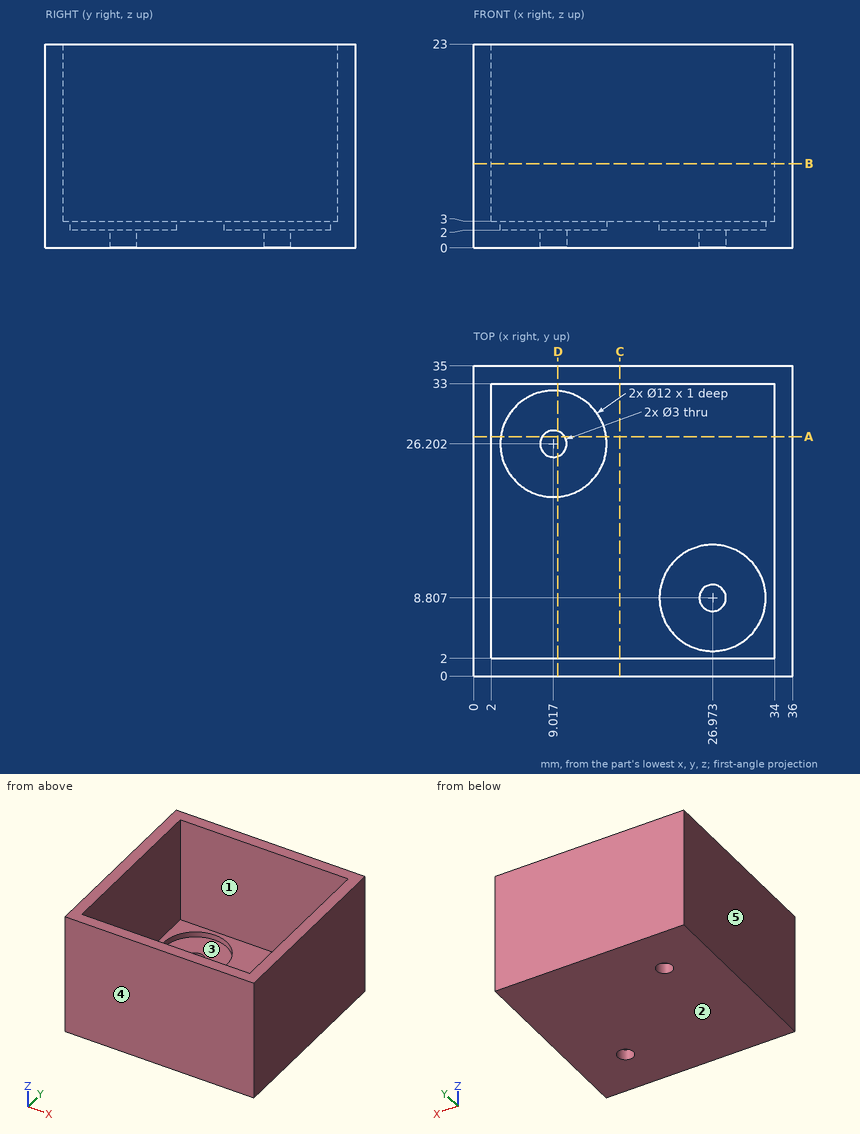
Geometry: see drawing. Coordinates: mm, zero at the bounding-box minimum. A direction names the side the tool comes from. Coordinates: 2 decimals unless noted, no trailing zeros. Loops run counter-clockwise (first coordinate to the right, second up) from the corner with the lowest first, then second, coordinate; pieces in that order, holes last. Notation, with made-up numbers: (40.5, -20.5) -> (69.5, -20.5) arc R34 ccw to (69.5, 10.5) -> close; hole circle Ø7 at (54, 79). An arc over 180 degrees is marked (long way). Write item = value, one per line. Start each with the question number.
Item 1: Cut plane B-B, the plane z = 9.5. Return loops of the section in (x, y), plus the area to 3 significant figures.
Item 2: Cut plane D-D, the plane x = 9.5. Return loops of the section in (y, z).
Item 3: Material intervals for line 1 (X direction, y = 30.5, z = 8.25); line 2 (Y direction, x = 15, z = 9.25); line 3 (Z direction, x = 30, y = 18.5), sorted ascending.
Item 4: Reachability of the marked faces 1 and 2 from +Z, -Z, +X, -X, +Y, -Y: full face, straight path, thin tool, end or side. Return the list, or none.
Item 5: First-contact query: P1, Ø9.5, axis at x = 18, y = 23, coming from the +Z side; P2, Ø12, axis at y = 10, z = 13, coming from the -X side; P3, Ø4, axis at x = 26.97, y = 8.81, coming from the +Z side. Flat tips, straight axial feed; report the tip coordinate or a pass-through.
Item 6: Mould query, pull axis Y, two halves, no side actions, for the marked faces 3, 4 and 5. Classes: pulls with the +Y half, pulls with the -Y half, needs draft (parallel to the pull), parting line crosses it, or undercut.
Item 7: Cut plane C-C, the plane x = 16.5. Return loops of the section in (y, z), plus the area to 3 significant figures.
Item 8: Cut plane A-A, the plane y = 27. Return loops of the section in (x, z) (1 decimal), plus the area to 3 significant figures.
Ans:
q1.outline = (0, 0) -> (36, 0) -> (36, 35) -> (0, 35) -> close; hole (2, 2) -> (34, 2) -> (34, 33) -> (2, 33) -> close
q1.area = 268 mm²
q2.outline = (0, 0) -> (24.78, 0) -> (24.78, 2) -> (20.22, 2) -> (20.22, 3) -> (2, 3) -> (2, 23) -> (0, 23) -> close; (27.62, 0) -> (35, 0) -> (35, 23) -> (33, 23) -> (33, 3) -> (32.18, 3) -> (32.18, 2) -> (27.62, 2) -> close
q3.line_1 = 0 to 2, 34 to 36
q3.line_2 = 0 to 2, 33 to 35
q3.line_3 = 0 to 3
q4.face_1 = +Z
q4.face_2 = -Z, +X, -X, +Y, -Y
q5.P1 = 3
q5.P2 = 0
q5.P3 = 2
q6.face_3 = undercut
q6.face_4 = pulls with the -Y half
q6.face_5 = needs draft
q7.outline = (0, 0) -> (35, 0) -> (35, 23) -> (33, 23) -> (33, 3) -> (2, 3) -> (2, 23) -> (0, 23) -> close
q7.area = 185 mm²
q8.outline = (0, 0) -> (7.7, 0) -> (7.7, 2) -> (3.1, 2) -> (3.1, 3) -> (2, 3) -> (2, 23) -> (0, 23) -> close; (10.3, 0) -> (36, 0) -> (36, 23) -> (34, 23) -> (34, 3) -> (15, 3) -> (15, 2) -> (10.3, 2) -> close
q8.area = 171 mm²
